The figure shows three views and two pictorial views of one solid part (mm, origin at its lowest corner). Answer the questions. Coordinates: 2 decimals unless noted, no trailing zeros. Order: outer loops, then holes, each group sorted by start corner. A loop starts at its lowest first (then second) coordinate and runs counter-clockwise, first axis right, second up.
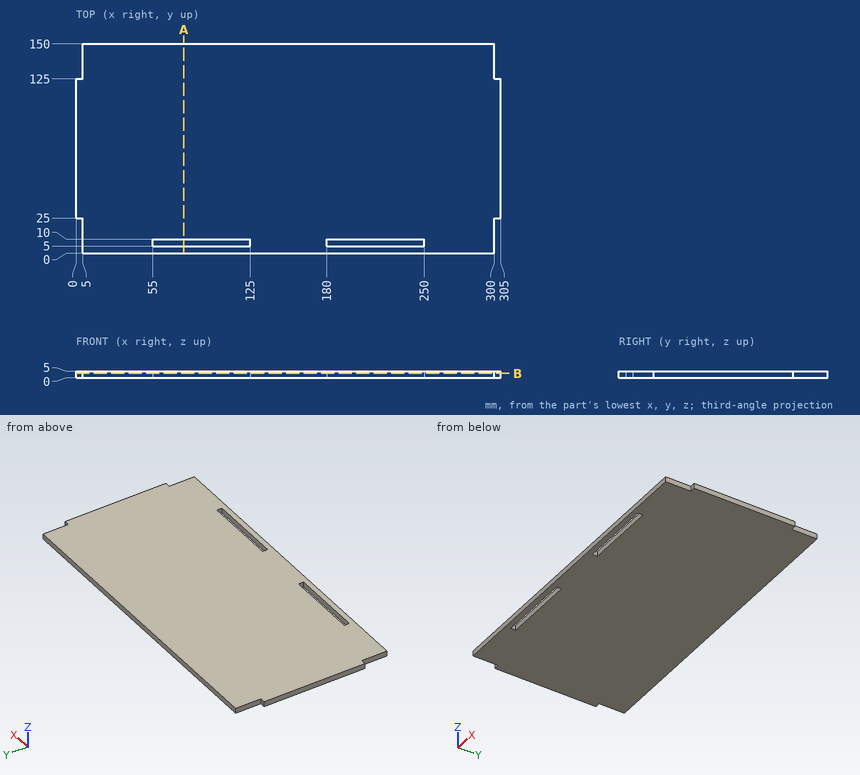
1) A cutting plane is placed at B-B, the plane z = 3.3. Write down the section's boundary in (x, y).
2) Each of these flat-tipped pins is pushed along its axis until it touches: P1, Ø1.5, axis at y = 136, z = 3, coming from the +X side; P2, Ø2.5, axis at y = 7.5, z = 3.5, coming from the -X side; P3, Ø1.5, axis at x = 3.5, z = 3.5, coming from the +Y side. Where does it stop, or does it pass through?
3) Straight lines are drawn through the part: probe 1 along Y at (x, z) = (207, 0.3); probe 2 along X at (y, z) = (144, 1.05). For each, find the intervals that lie inside material, in ascending order.
4) A cutting plane is placed at A-A, the plane x = 77.5. Write down the section's boundary in (y, z).
Working result:
1. outline: (0, 25) - (5, 25) - (5, 0) - (300, 0) - (300, 25) - (305, 25) - (305, 125) - (300, 125) - (300, 150) - (5, 150) - (5, 125) - (0, 125) - close; hole (55, 5) - (125, 5) - (125, 10) - (55, 10) - close; hole (180, 5) - (250, 5) - (250, 10) - (180, 10) - close
2. P1: stops at x = 300
2. P2: stops at x = 5
2. P3: stops at y = 125
3. probe 1: y = 0 to 5, 10 to 150
3. probe 2: x = 5 to 300
4. outline: (0, 0) - (5, 0) - (5, 5) - (0, 5) - close; (10, 0) - (150, 0) - (150, 5) - (10, 5) - close
